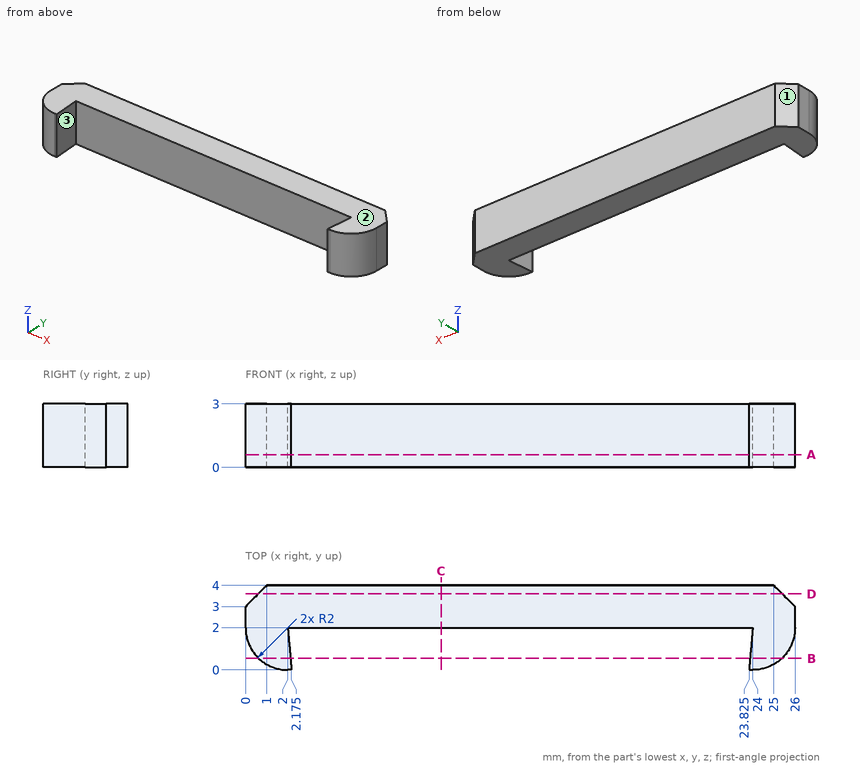
Design review of the part shown in the three views and the two pictorial views. Dimensions are in mm from the part's minimum x, y and z. Give positions to 0.01 mm unless a question says otherwise; leave off trailing zeros. Write each loop counter-clockwise with the first axis right and the second up, starting at its lowest first coordinate (ties: lowest second). Pieces come first, ordered by that corner, then holes.
Item 1: The part is to be moulded in two halves that separate along Y. For the marked faces 1, 2 and 3, say which applies: +Y half, -Y half, draft (parallel to the pull), parting line (faces both ways), or undercut.
Item 2: Wall thickness on probe 1 along Y at (x, z) = (6, 1.6); probe 2 along X at (y, z) = (1.1, 1.9); probe 3 along X at (y, z) = (1.75, 2.05): over which ranges is each line inside the solid? List them lowest first.
Item 3: Take a section at B-B (y = 0.55). Give the boundary of the cut face in (x, z), and give its area (3 significant figures).
Item 4: Insertion check: P1, Ø0.9, axis at x = 9.5, z = 1.5, coming from the -Y side. The pin has a flat end and moves straight along its axis. Give the tip position at first contact, or say it passes through.
Item 5: Take a section at A-A (z = 0.6). Give the boundary of the cut face in (x, y) (3 decimals).
Item 6: Take a section at C-C (x = 9.25). Give the boundary of the cut face in (y, z), and give its area (3 significant figures).
Item 7: Take a section at D-D (y = 3.6). Give the boundary of the cut face in (x, z), and give its area (3 significant figures).
Established:
1. face 1: +Y half
1. face 2: draft
1. face 3: undercut
2. probe 1: y = 2 to 4
2. probe 2: x = 0.21 to 2.08, 23.92 to 25.79
2. probe 3: x = 0.02 to 2.02, 23.98 to 25.98
3. outline: (0.62, 0) - (2.13, 0) - (2.13, 3) - (0.62, 3) - close; (23.87, 0) - (25.38, 0) - (25.38, 3) - (23.87, 3) - close
3. area: 9.03 mm2
4. P1: stops at y = 2
5. outline: (0, 2) arc R2 ccw to (2, 0) - (2.175, 0) - (2, 2) - (24, 2) - (23.825, 0) - (24, 0) arc R2 ccw to (26, 2) - (26, 3) - (25, 4) - (1, 4) - (0, 3) - close
6. outline: (2, 0) - (4, 0) - (4, 3) - (2, 3) - close
6. area: 6.00 mm2
7. outline: (0.6, 0) - (25.4, 0) - (25.4, 3) - (0.6, 3) - close
7. area: 74.4 mm2
